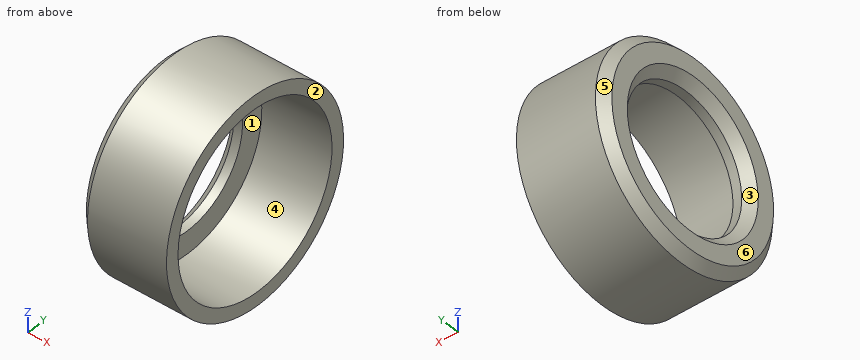
```python
from build123d import *

# Parameters (mm, degrees)
F3_SIZE = 2
F4_SIZE = 2


with BuildPart() as f2:
    # F0 (on Front) → F2 (revolve)
    with BuildSketch(Plane.XZ):
        Polygon((8.34782, 20), (8.34782, 15), (12.34782, 15), (12.34782, 20), (28.34782, 20), (28.34782, 23), (8.34782, 23), align=None)
    revolve(axis=Axis((1.375284, 0, 0), (1, 0, 0)))

    # F3
    f3_edges = [f2.edges().sort_by_distance(p)[0] for p in [
        (8.34782, 0, -23),
    ]]
    chamfer(f3_edges, length=F3_SIZE)

    # F4
    f4_edges = [f2.edges().sort_by_distance(p)[0] for p in [
        (8.34782, 0, -15),
    ]]
    chamfer(f4_edges, length=F4_SIZE)


solid = f2.part
```
Work out the finished part from the listing and answer in its coordinate system (mm). Face numbers are marked on the shaded views. A direction names the side the tool comes from. Give positions to 0.01 mm unless a question says otherwise; leave off trailing zeros. Order: outer loops, then holes, each group sorted by start corner. A loop starts at its lowest first (then second) coordinate and runs counter-clockwise, first axis right, second up. Notation, with made-up numbers: (22, 44) -> (72, 44) arc R19 ccw to (72, 80) -> close; hole circle Ø3 at (34.25, -32). An arc over 180 degrees is marked (long way). Answer as CSV lines item,"result". Start each with the question number.
(1) Each of these flat-tipped pins is pushed along its axis until it touches: pin 1 Ø5 at (x, y) = (14, -4.5) entering from -Z; pin 2 Ø2 at (x, y) = (21.5, 12) entering from +Z; pin 3 Ø6 at (x, z) = (22.5, -11.5) entering from +Y; pin 4 Ø1 at (y, z) = (-0.5, 13) entering from -X. Where does it stop, or does it pass through?
(2) For a pull along Y with two mould halves and no side action, classify the marked faces 3, 4, 5 and 6 as released by +Y, released by -Y, zero draft, split by the parting line, or undercut.
(3) Section A-A, the plane z = 0 is taken. Write down the section's boundary in (x, y).
(4) Which of the six approach directions +Z, -Z, +X, -X, +Y, -Y give full straight-line access (tool end or side, diameter ignored) to the marked faces 1 and 2?
(5) Consider line 1 along Z through (x, y) = (11.2, 0); line 2 along Y through (x, z) = (15.5, 0). Determine where each line is inside the solid, lowest interval first.
(6) Section C-C, the plane x = 26.75 is taken. Write down the section's boundary in (y, z).
Entries:
1,pin 1,"z = -22.91"
1,pin 2,"z = 20.2"
1,pin 3,"y = 21.37"
1,pin 4,"through"
2,face 3,"undercut"
2,face 4,"undercut"
2,face 5,"split by the parting line"
2,face 6,"zero draft"
3,outline,"(8.35, -21) -> (10.35, -23) -> (28.35, -23) -> (28.35, -20) -> (12.35, -20) -> (12.35, -15) -> (10.35, -15) -> (8.35, -17) -> close; (8.35, 17) -> (10.35, 15) -> (12.35, 15) -> (12.35, 20) -> (28.35, 20) -> (28.35, 23) -> (10.35, 23) -> (8.35, 21) -> close"
4,face 1,"+X"
4,face 2,"+Z, -Z, +X, +Y, -Y"
5,line 1,"-23 to -15, 15 to 23"
5,line 2,"-23 to -20, 20 to 23"
6,outline,"circle Ø46 at (0, 0); hole circle Ø40 at (0, 0)"
